from build123d import *

# Parameters (mm, degrees)
SKETCH1_R                       = 25.4
BOSS_EXTRUDE1_DEPTH             = 12.7
SKETCH9_R                       = 14.605
BOSS_EXTRUDE2_DEPTH             = 38.1
F_10_24_TAPPED_HOLE1_D          = 3.9878
F_8_4_8_4_DIAMETER_HOLE2_D      = 8.4
F_10_0_10_DIAMETER_HOLE1_D      = 10
F_10_0_10_DIAMETER_HOLE1_DEPTH  = 10.16
F_10_0_10_DIAMETER_HOLE1_TIP    = 3.004303095
F_3_4_0_75_DIAMETER_HOLE1_D     = 19.05
F_3_4_0_75_DIAMETER_HOLE1_DEPTH = 22.86
F_3_4_0_75_DIAMETER_HOLE1_TIP   = 5.723197396


with BuildPart() as part:
    # Sketch1 → Boss-Extrude1 (new body)
    with BuildSketch(Plane.XY):
        Circle(SKETCH1_R)
    extrude(amount=-BOSS_EXTRUDE1_DEPTH)

    # Sketch9 → Boss-Extrude2 (add)
    with BuildSketch(Plane.XY):
        Circle(SKETCH9_R)
    extrude(amount=-BOSS_EXTRUDE2_DEPTH)

    # #10-24 Tapped Hole1 (through all)
    with Locations(Plane(origin=(0, 0, -12.7), x_dir=(-1, 0, 0), z_dir=(0, 0, -1))):
        with Locations((0, 19.05), (-16.497783942, -9.525), (16.497783942, -9.525)):
            Hole(F_10_24_TAPPED_HOLE1_D / 2)

    # Ø8.4 (8.4) Diameter Hole2 (through all)
    with Locations(Plane(origin=(0, 0, -38.1), x_dir=(-1, 0, 0), z_dir=(0, 0, -1))):
        with Locations((0, 0)):
            Hole(F_8_4_8_4_DIAMETER_HOLE2_D / 2)

    # Ø10.0 (10) Diameter Hole1
    with Locations(Plane(origin=(0, 0, -38.1), x_dir=(-1, 0, 0), z_dir=(0, 0, -1))):
        with Locations((0, 0)):
            Hole(F_10_0_10_DIAMETER_HOLE1_D / 2, depth=F_10_0_10_DIAMETER_HOLE1_DEPTH)
            with Locations((0, 0, -(F_10_0_10_DIAMETER_HOLE1_DEPTH + F_10_0_10_DIAMETER_HOLE1_TIP / 2))):  # 118° drill point
                Cone(0, F_10_0_10_DIAMETER_HOLE1_D / 2, F_10_0_10_DIAMETER_HOLE1_TIP, mode=Mode.SUBTRACT)

    # 3/4 (0.75) Diameter Hole1
    with Locations(Plane.XY):
        with Locations((0, 0)):
            Hole(F_3_4_0_75_DIAMETER_HOLE1_D / 2, depth=F_3_4_0_75_DIAMETER_HOLE1_DEPTH)
            with Locations((0, 0, -(F_3_4_0_75_DIAMETER_HOLE1_DEPTH + F_3_4_0_75_DIAMETER_HOLE1_TIP / 2))):  # 118° drill point
                Cone(0, F_3_4_0_75_DIAMETER_HOLE1_D / 2, F_3_4_0_75_DIAMETER_HOLE1_TIP, mode=Mode.SUBTRACT)


solid = part.part
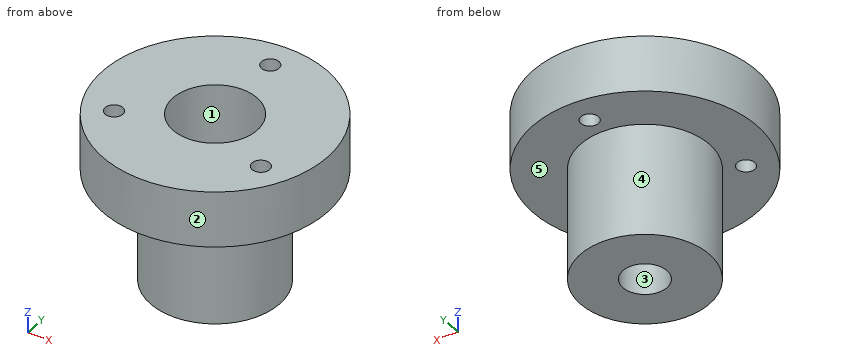
Read the model definition and answer for the solid it produces. Units are mm, in the model's axes. Face numbers are marked on the shaded views. A direction names the side the tool comes from. Coordinates: 2 decimals unless noted, no trailing zeros. Order: outer loops, then holes, each group sorted by start corner. A loop starts at its lowest first (then second) coordinate and runs counter-clockwise, first axis right, second up. Notation, with made-up numbers: M 69,86.5 L 117,86.5 A36 cw 117,123.5 Z; hole C 1,6 d7. An arc over 180 degrees is marked long. Put each result on its own line as item: value. Start each with the question number.
Item 1: Section D-D, the plane z = -3 is taken. Determine the outline of the cut face in (x, y) (3 decimals).
Item 2: Section B-B, the plane x = 0 is taken. Determine the outline of the cut face in (y, z) (3 decimals), plus the area to 3 significant figures.
Item 3: Section C-C, the plane z = -20.5 is taken. Determine the outline of the cut face in (x, y) (3 decimals), plus the area to 3 significant figures.
Item 4: Section A-A, the plane y = 0 is taken. Determine the outline of the cut face in (x, z) (3 decimals).
Item 5: For the marked faces 1 and 2, determine the directions among +Z, -Z, +X, -X, +Y, -Y from which every point of the face is accessible in a straight line to the end or side of a thin tool.
Item 6: The mould has two halves that part along X. Classify the marked faces 3, 4 and 5: +X half, -X half, draft (parallel to the pull), parting line (faces both ways), or undercut.
Item 7: Consider probe 1 along Y at (x, z) = (0, -5.5) (3 decimals); probe 2 along Y at (x, z) = (0, -27.05) (3 decimals); probe 3 along X at (y, z) = (0.5, -13). Determine where each line is inside the solid, lowest interval first. Write a range as [from, to].
Item 8: Given pin 1 Ø2 at (x, z) = (-5.5, -24.5) entering from -Y; pin 2 Ø6 at (x, y) = (-13.5, -18) entering from +Z; pin 3 Ø4 at (x, z) = (-8.5, -11.5) entering from -Y; pin 4 Ø1.5 at (y, z) = (3, -25) entering from -X, each flat-ended and moving along its own axis, determine where each tip first touches the part or whether it passes through.
Computed:
1. outline: C 0,0 d50.8; hole C -16.498,-9.525 d3.988; hole C 0,0 d19.05; hole C 0,19.05 d3.988; hole C 16.498,-9.525 d3.988
2. outline: M -25.4,-12.7 L -14.605,-12.7 L -14.605,-38.1 L -5,-38.1 L -5,-27.94 L -4.2,-27.459 L -4.2,-26.06 L -9.525,-22.86 L -9.525,0 L -25.4,0 Z; M 4.2,-27.459 L 5,-27.94 L 5,-38.1 L 14.605,-38.1 L 14.605,-12.7 L 17.056,-12.7 L 17.056,0 L 9.525,0 L 9.525,-22.86 L 4.2,-26.06 Z; M 21.044,-12.7 L 25.4,-12.7 L 25.4,0 L 21.044,0 Z
2. area: 739 mm2
3. outline: C 0,0 d29.21; hole C 0,0 d19.05
3. area: 385 mm2
4. outline: M -25.4,-12.7 L -14.605,-12.7 L -14.605,-38.1 L -5,-38.1 L -5,-27.94 L -4.2,-27.459 L -4.2,-26.06 L -9.525,-22.86 L -9.525,0 L -25.4,0 Z; M 4.2,-27.459 L 5,-27.94 L 5,-38.1 L 14.605,-38.1 L 14.605,-12.7 L 25.4,-12.7 L 25.4,0 L 9.525,0 L 9.525,-22.86 L 4.2,-26.06 Z
5. face 1: +Z
5. face 2: +Z, -Z
6. face 3: undercut
6. face 4: parting line
6. face 5: draft
7. probe 1: y = [-25.4, -9.525], [9.525, 17.056], [21.044, 25.4]
7. probe 2: y = [-14.605, -4.2], [4.2, 14.605]
7. probe 3: x = [-14.6, -9.51], [9.51, 14.6]
8. pin 1: stops at y = -13.89
8. pin 2: stops at z = 0
8. pin 3: stops at y = -24.55
8. pin 4: stops at x = -14.43
